```python
from build123d import *

# Parameters (mm, degrees)
F0_W      = 117.348
F0_H      = 62.992
F1_DEPTH  = 50.8
F2_W      = 41.148
F2_H      = 18.796
F3_DEPTH  = 50.801
F4_W      = 60.452
F4_H      = 12.7
F5_DEPTH  = 50.801
F6_W      = 35.052
F6_H      = 12.7124151424
F7_DEPTH  = 76.201
F8_W      = 15.7580270052
F8_H      = 31.496
F9_DEPTH  = 117.349
F10_W     = 15.7580270052
F10_H     = 6.0835848576
F11_DEPTH = 76.201
F12_W     = 15.748
F12_H     = 12.7
F13_DEPTH = 117.349
F14_R     = 9.525
F15_DEPTH = 35.0429729948


with BuildPart() as f1:
    # F0 (on Front) → F1 (new body)
    with BuildSketch(Plane.XZ):
        Rectangle(F0_W, F0_H)
    extrude(amount=F1_DEPTH)

    # F2 (on face) → F3 (cut, through all)
    with BuildSketch(Plane.XZ.offset(50.8)):
        with Locations((38.1, 22.098)):
            Rectangle(F2_W, F2_H)
    extrude(amount=-F3_DEPTH, mode=Mode.SUBTRACT)

    # F4 (on face) → F5 (cut, through all)
    with BuildSketch(Plane.XZ.offset(50.8)):
        with Locations((-28.448, -25.146)):
            Rectangle(F4_W, F4_H)
    extrude(amount=-F5_DEPTH, mode=Mode.SUBTRACT)

    # F6 (on face) → F7 (cut, through all)
    with BuildSketch(Plane.YZ.offset(17.526)):
        with Locations((-33.274, 25.1397924288)):
            Rectangle(F6_W, F6_H)
    extrude(amount=-F7_DEPTH, mode=Mode.SUBTRACT)

    # F8 (on face) → F9 (cut, through all)
    with BuildSketch(Plane.YZ.offset(58.674)):
        with Locations((-42.9209864974, -3.048)):
            Rectangle(F8_W, F8_H)
    extrude(amount=-F9_DEPTH, mode=Mode.SUBTRACT)

    # F10 (on face) → F11 (cut, through all)
    with BuildSketch(Plane.YZ.offset(17.526)):
        with Locations((-42.9209864974, 15.7417924288)):
            Rectangle(F10_W, F10_H)
    extrude(amount=-F11_DEPTH, mode=Mode.SUBTRACT)

    # F12 (on face) → F13 (cut, through all)
    with BuildSketch(Plane.YZ.offset(58.674)):
        with Locations((-7.874, -25.146)):
            Rectangle(F12_W, F12_H)
    extrude(amount=-F13_DEPTH, mode=Mode.SUBTRACT)

    # F14 (on face) → F15 (cut, through all)
    with BuildSketch(Plane.XZ.offset(35.0419729948)):
        with Locations((-26.67, 0)):
            Circle(F14_R)
    extrude(amount=-F15_DEPTH, mode=Mode.SUBTRACT)


solid = f1.part
```
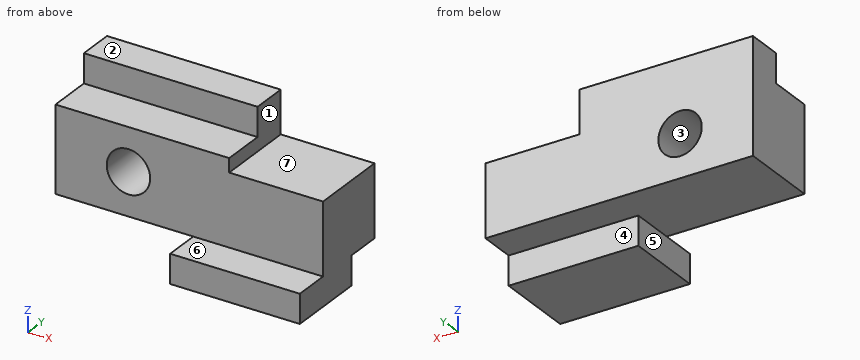
Source: CAD feature listing. Evaluate the final solid. Frame: model axes, mm. Face numbers are marked on the shaded views. A direction names the side the tool comes from. Coordinates: 2 decimals unless noted, no trailing zeros. Loops run counter-clockwise (first coordinate to the right, second up) from the corner with the lowest first, then second, coordinate; pieces in that order, holes last. Notation, with made-up numbers: (83, 69) -> (110, 69) arc R27 ccw to (110, 107) -> close; hole circle Ø9 at (79, -35). An arc over 180 degrees is marked (long way). One line per item, written item: value. Start each with the question number.
Q1. Section query C-C, the plane y = -10. Return the cut outline in (x, z) (3 decimals).
Q2. Set-up query: the marked faces 4, 5, 6 and 7. Return all of +Z, -Z, +X, -X, +Y, -Y with unobstructed straight access to the full face (end or side cutting, diameter ignored); none if empty.
Q3. Line query: line 1 along Z through (x, y) = (-26.67, -19.5) (3 decimals); line 2 along Z through (x, y) = (-26, -8); line 3 along Y through (x, z) = (34, -7). Output: solid intervals per line, ascending.
Q4. Section query D-D, the plane x = 26.5. Return the cut outline in (y, z).
Q5. Mould query, pull axis Z, two halves, no side actions, for the marked faces 1, 2 and 3. Classes: pulls with the +Z half, pulls with the -Z half, needs draft (parallel to the pull), parting line crosses it, or undercut.
Q6. Section query B-B, the plane x = -26.67. Return the cut outline in (y, z) (3 decimals).
Q7. Section query A-A, the plane z = 0. Return the cut outline in (x, y) (3 decimals).
Q8. Contact query for flat-ended pins moving along their axis: P1, Ø8, axis at x = -31.5, z = 15, coming from the -Y side; P2, Ø15, axis at y = -24.5, z = 23.5, coming from the +X side; P3, Ø4, axis at x = -14.5, z = 23, coming from the -Y side. Output: stop coordinate, or through.
Results:
1. outline: (-58.674, -18.796) -> (58.674, -18.796) -> (58.674, 12.7) -> (17.526, 12.7) -> (17.526, 31.496) -> (-58.674, 31.496) -> close; hole circle Ø19.05 at (-26.67, 0)
2. face 4: -Z, +X, -X, +Y
2. face 5: -Z, -X, +Y, -Y
2. face 6: +Z, +X, -X, -Y
2. face 7: +Z, +X, +Y, -Y
3. line 1: -18.796 to -9.525, 9.525 to 18.784
3. line 2: -18.8 to -9.5, 9.5 to 31.5
3. line 3: -35.04 to 0
4. outline: (-50.8, -31.5) -> (-15.75, -31.5) -> (-15.75, -18.8) -> (0, -18.8) -> (0, 12.7) -> (-35.04, 12.7) -> (-35.04, -18.8) -> (-50.8, -18.8) -> close
5. face 1: needs draft
5. face 2: pulls with the +Z half
5. face 3: undercut
6. outline: (-35.042, -18.796) -> (0, -18.796) -> (0, -9.525) -> (-35.042, -9.525) -> close; (-35.042, 9.525) -> (0, 9.525) -> (0, 31.496) -> (-15.748, 31.496) -> (-15.748, 18.784) -> (-35.042, 18.784) -> close
7. outline: (-58.674, -35.042) -> (-36.195, -35.042) -> (-36.195, 0) -> (-58.674, 0) -> close; (-17.145, -35.042) -> (58.674, -35.042) -> (58.674, 0) -> (-17.145, 0) -> close
8. P1: y = -35.04
8. P2: x = 17.53
8. P3: y = -15.75
